```python
from build123d import *

# Parameters (mm, degrees)
BOSS_EXTRUDE2_DEPTH = 38.1
SKETCH24_W          = 13.462
SKETCH24_H          = 6.242787019
FILLET16_R          = 3.81
CUT_EXTRUDE3_DEPTH  = 11.1125
SKETCH101_R         = 2.54
CUT_EXTRUDE4_DEPTH  = 17.78
SKETCH102_W         = 10.16
SKETCH102_H         = 1.27
CHAMFER1_SIZE       = 12.7
FILLET17_R          = 1.5875


with BuildPart() as part:
    # Sketch7 → Boss-Extrude2 (new body)
    with BuildSketch(Plane(origin=(0, 0, 0), x_dir=(1, 0, 0), z_dir=(0, 1, 0))):
        Polygon((0, 0), (11.1125, 0), (20.6375, -9.525), (20.6375, -23.8125), (-23.8125, -23.8125), align=None)
    boss_extrude2 = extrude(amount=BOSS_EXTRUDE2_DEPTH)

    # Sketch24 → Port Manifold (revolve, cut)
    with BuildSketch(Plane.ZY.offset(-4.7625)):
        with Locations((17.0815, 18.99639351)):
            Rectangle(SKETCH24_W, SKETCH24_H)
    port_manifold = revolve(axis=Axis((4.7625, 15.875, 10.3505), (0, 0, 1)), mode=Mode.SUBTRACT)

    # Mirror6: Boss-Extrude2, Port Manifold across Plane1
    add(boss_extrude2.mirror(Plane(origin=(0, 0, 0), x_dir=(0.707106781, 0, -0.707106781), z_dir=(0.707106781, 0, 0.707106781))))
    add(port_manifold.mirror(Plane(origin=(0, 0, 0), x_dir=(0.707106781, 0, -0.707106781), z_dir=(0.707106781, 0, 0.707106781))), mode=Mode.SUBTRACT)

    # Fillet16
    fillet16_edges = [part.edges().sort_by_distance(p)[0] for p in [
        (20.6375, 38.1, 16.66875),
        (-16.66875, 38.1, -20.6375),
    ]]
    fillet(fillet16_edges, radius=FILLET16_R)

    # Sketch93 → Cut-Extrude3 (cut)
    with BuildSketch(Plane(origin=(0, 38.1, 0), x_dir=(1, 0, 0), z_dir=(0, 1, 0))):
        with BuildLine():
            Line((-23.8125, -23.8125), (-1.5875, -23.8125))
            Line((-1.5875, -23.8125), (-1.5875, -6.35))
            ThreePointArc((-1.5875, -6.35), (-2.982403955, -2.982403955), (-6.35, -1.5875))
            Line((-6.35, -1.5875), (-23.8125, -1.5875))
            Line((-23.8125, -1.5875), (-23.8125, -23.8125))
        make_face()
    extrude(amount=-CUT_EXTRUDE3_DEPTH, mode=Mode.SUBTRACT)

    # Sketch101 → Cut-Extrude4 (cut)
    with BuildSketch(Plane.XZ):
        with Locations((-9.8425, 9.8425)):
            Circle(SKETCH101_R)
    extrude(amount=-CUT_EXTRUDE4_DEPTH, mode=Mode.SUBTRACT)

    # Sketch102 → Cut-Revolve1 (revolve, cut)
    with BuildSketch(Plane(origin=(0, 15.875, 0), x_dir=(1, 0, 0), z_dir=(0, 1, 0))):
        with Locations((-5.5245, -9.9695)):
            Rectangle(SKETCH102_W, SKETCH102_H)
    cut_revolve1 = revolve(axis=Axis((-0.4445, 15.875, 9.3345), (-1, 0, 0)), mode=Mode.SUBTRACT)

    # Mirror10: Cut-Revolve1 across plane
    add(cut_revolve1.mirror(Plane(origin=(0, 0, 0), x_dir=(-0.707106781, 0, 0.707106781), z_dir=(0.707106781, 0, 0.707106781))), mode=Mode.SUBTRACT)

    # Chamfer1
    chamfer1_edges = [part.edges().sort_by_distance(p)[0] for p in [
        (-23.8125, 13.49375, 23.8125),
    ]]
    chamfer(chamfer1_edges, length=CHAMFER1_SIZE)

    # Fillet17
    fillet17_edges = [part.edges().sort_by_distance(p)[0] for p in [
        (0, 19.05, 0),
    ]]
    fillet(fillet17_edges, radius=FILLET17_R)


solid = part.part
```
Can you work these out from the model? Positions are in its coordinate system, mm. A direction names the side the tool comes from. Round coordinates to 2 decimals unless told otherwise and drop trailing zeros. Loops run counter-clockwise (first coordinate to the right, second up) from the corner with the lowest first, then second, coordinate; pieces in that order, holes last. Notation, with made-up numbers: M 41,30.5 L 99,30.5 A30 cw 99,69.5 Z; hole C 3.25,80.5 d10. An arc over 180 degrees is marked long. Write item = value, one per line. Start each with the question number.
(1) Suppose I cut it at A-A on z = 14.5. Write out the boundary of the cut face in (x, y) (1 decimal), plus the area to 3 significant figures.
(2) Which directions (+Z, -Z, +X, -X, +Y, -Y) give clear straight access to the entire face, cutting with the end or side of a thin tool? Please do faces 1 (the face through (-17.18, 18.76, -10.3)), 2 (the face through (-11.715, 8.766, 11.559)), 3 (the face through (-1.588, 33, 15)), 4 (the face through (0, 19, -6)), 5 (the face through (-9, 16, 0.444)).
(3) Suppose I cut it at C-C on x = -15. Write out the boundary of the cut face in (y, z) (1 decimal), plus the area to 3 significant figures.
(4) I'm going to push flat-ended pins straight in: P1, Ø12, axis at x = -17.5, y = 33.5, coming from the +Z side; P2, Ø3, axis at y = 12, z = -2, coming from the +X side; P3, Ø3.5, axis at x = 3.5, y = 16.5, coming from the +Z side; P4, Ø12, axis at y = 31, z = 13, coming from the -X side. Where does each tip first touch, or does it pass through?
(5) Suppose I cut it at B-B on y = 24.5. Write out the boundary of the cut face in (x, z) (1 decimal), plus the area to 3 significant figures.
(6) If we mould it in two halves opening along Z, with no side actions, what happens to faces 6 (the face through (5, 16, 10.35)), 7 (the face through (-10.351, 16, -5)), 8 (the face through (-23.813, 19, -12)), 9 (the face through (-4.7, 18.78, -15.81))? For each: released by +Z, released by -Z, zero draft, split by the parting line, or undercut.
(7) I need wall thicknesses on line 1 along Z through (x, y) = (-11.5, 17) (1 decimal); line 2 along Z through (x, y) = (-12, 10.5) (1 decimal); line 3 along X through (y, z) = (24, -7). Which ranges of each line are inside material? Lowest first, please.
(8) Suppose I cut it at D-D on x = 6.5. Write out the boundary of the cut face in (y, z).
Answer block:
q1.outline = M -20.4,0 L 20.6,0 L 20.6,34.3 A3.8 ccw 16.8,38.1 L -1.6,38.1 L -1.6,27 L -20.4,27 Z; hole C 4.8,15.9 d12.5
q1.area = 1,230 mm²
q2.face_1 = -X
q2.face_2 = -Y
q2.face_3 = +Z, -X, +Y
q2.face_4 = -Z, +X, +Y, -Y
q2.face_5 = none
q3.outline = M 0,-20.6 L 34.3,-20.6 A3.8 ccw 38.1,-16.8 L 38.1,1.6 L 27,1.6 L 27,19.9 L 0,19.9 Z; hole C 15.9,-4.8 d12.5
q3.area = 1,220 mm²
q4.P1 = 1.59
q4.P2 = 0.43
q4.P3 = 10.35
q4.P4 = -23.81
q5.outline = M -23.8,-20.6 L -9.5,-20.6 L 0,-11.1 L 0,-1.6 A1.6 cw 1.6,0 L 11.1,0 L 20.6,9.5 L 20.6,23.8 L -11.1,23.8 L -23.8,11.1 Z
q5.area = 1,380 mm²
q6.face_6 = released by +Z
q6.face_7 = undercut
q6.face_8 = zero draft
q6.face_9 = released by -Z
q7.line_1 = -20.6 to -10.9, 1.4 to 7.9, 11.8 to 23.4
q7.line_2 = -20.6 to -7.9, -1.6 to 8.5, 11.2 to 22.9
q7.line_3 = -23.81 to 0
q8.outline = M 0,0 L 38.1,0 L 38.1,23.81 L 21.87,23.81 L 21.87,10.35 L 9.88,10.35 L 9.88,23.81 L 0,23.81 Z
